Answer from the drawing. Dimensions are ordinates in mm from the lowest x, y and z of the part. A direction names the side the tool comes from. Coordinates: 2 decimals unless noted, no trailing zeros. Loops run counter-clockwise (first coordinate to the right, second up) from the corner with the lowest first, then second, coordinate; pieces in that order, holes last. Notation, with made-up numbers: (-21.75, 39.5) -> (-9.75, 39.5) arc R20 ccw to (-9.75, 62.5) -> close; hole circle Ø7 at (-32.75, 18.25). An arc over 180 degrees is marked (long way). Use a Markdown table: item, result.
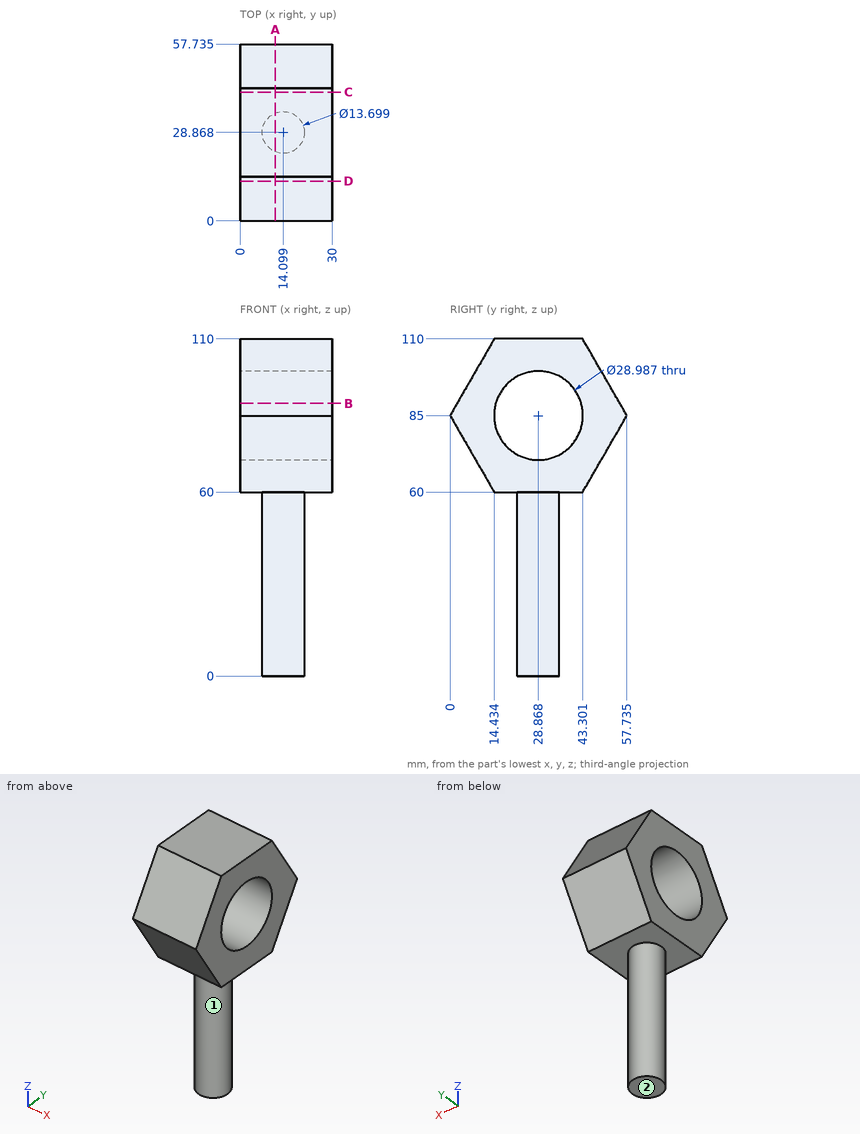
Q1. Section C-C on y = 42 is taken. Determine the outline of the cut face in (x, z), and give its area (3 significant figures).
Solved:
| item | result |
|---|---|
| outline | (0, 60) -> (30, 60) -> (30, 78.87) -> (0, 78.87) -> close; (0, 91.13) -> (30, 91.13) -> (30, 110) -> (0, 110) -> close |
| area | 1,130 mm² |
Q2. Consider line 1 (Y direction, x = 9, z = 85) (1 decimal); line 2 (Y direction, x = 14.5, z = 54.5) (1 decimal); line 3 (Z direction, x = 12, y = 37) (1 decimal). Determine where each line is inside the solid, lowest interval first. Write a range as [from, to].
Solved:
| item | result |
|---|---|
| line 1 | [0, 14.4], [43.4, 57.7] |
| line 2 | [22, 35.7] |
| line 3 | [60, 73], [97, 110] |
Q3. Given pin 1 Ø8 at (y, z) = (51, 66.5) entering from +X; pin 2 Ø6 at (x, y) = (19.5, 16) entering from -Z; pin 3 Ø2 at (x, z) = (13, 64.5) entering from +Y; pin 4 Ø5 at (y, z) = (25, 95) entering from +X, each flat-ended and moving along its own axis, determine where each tip first touches the part or whether it passes through.
Solved:
| item | result |
|---|---|
| pin 1 | x = 30 |
| pin 2 | z = 60 |
| pin 3 | y = 46.48 |
| pin 4 | through |
Q4. Section B-B on z = 89 is taken. Determine the outline of the cut face in (x, y) (1 decimal).
Solved:
| item | result |
|---|---|
| outline | (0, 2.3) -> (30, 2.3) -> (30, 14.9) -> (0, 14.9) -> close; (0, 42.8) -> (30, 42.8) -> (30, 55.4) -> (0, 55.4) -> close |
Q5. For the marked faces 1 and 2, determine the directions among +Z, -Z, +X, -X, +Y, -Y from which every point of the face is accessible in a straight line to the end or side of a thin tool.
Solved:
| item | result |
|---|---|
| face 1 | -Z |
| face 2 | -Z, +X, -X, +Y, -Y |
Q6. Section D-D on y = 13 is taken. Determine the outline of the cut face in (x, z).
Solved:
| item | result |
|---|---|
| outline | (0, 62.48) -> (30, 62.48) -> (30, 107.52) -> (0, 107.52) -> close |
Q7. Section A-A on x = 11.5 is taken. Determine the outline of the cut face in (y, z) (1 decimal).
Solved:
| item | result |
|---|---|
| outline | (0, 85) -> (14.4, 60) -> (22.5, 60) -> (22.5, 0) -> (35.2, 0) -> (35.2, 60) -> (43.3, 60) -> (57.7, 85) -> (43.3, 110) -> (14.4, 110) -> close; hole circle Ø29 at (28.9, 85) |
